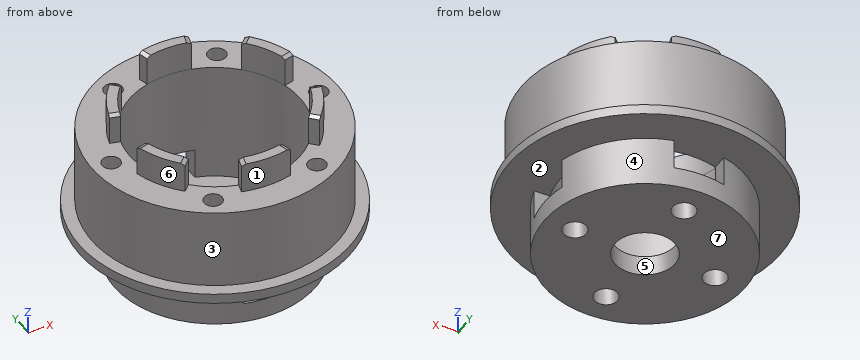
```python
from build123d import *
from OCP.BRepFilletAPI import BRepFilletAPI_MakeChamfer

# Parameters (mm, degrees)
SKETCH_1_R               = 10
EXTRUDE_1_DEPTH          = 2
SKETCH_2_R               = 10
SKETCH_2_R_2             = 8.5
EXTRUDE_2_DEPTH          = 3
SKETCH_4_R               = 13.5
SKETCH_4_R_2             = 8.5
EXTRUDE_3_DEPTH          = 1
SKETCH_5_R               = 12.25
SKETCH_5_R_2             = 8.5
EXTRUDE_4_DEPTH          = 8
SKETCH_6_R               = 0.9
CUT_EXTRUDE_1_DEPTH      = 8
SKETCH_7_R               = 3
SKETCH_7_R_2             = 1.15
CUT_EXTRUDE_2_DEPTH      = 24.674881204
CUT_EXTRUDE_3_DEPTH      = 24.674881204
CUT_EXTRUDE_3_DEPTH_BACK = 24.674881204
SKETCH_8_W               = 5
SKETCH_8_H               = 3
CUT_EXTRUDE_4_DEPTH      = 24.674881204
CUT_EXTRUDE_4_DEPTH_BACK = 24.674881204
SKETCH_9_W               = 3
SKETCH_9_H               = 5
EXTRUDE_5_DEPTH          = 3
CHAMFER_1_SIZE           = 0.2
CHAMFER_1_SIZE2          = 0.410060768


with BuildPart() as part:
    # 스케치1 → 보스-돌출1 (new body)
    with BuildSketch(Plane.XY):
        Circle(SKETCH_1_R)
    extrude(amount=EXTRUDE_1_DEPTH)

    # 스케치2 → 보스-돌출2 (add)
    with BuildSketch(Plane.XY.offset(2)):
        Circle(SKETCH_2_R)
        Circle(SKETCH_2_R_2, mode=Mode.SUBTRACT)
    extrude(amount=EXTRUDE_2_DEPTH)

    # 스케치4 → 보스-돌출3 (add)
    with BuildSketch(Plane.XY.offset(5)):
        Circle(SKETCH_4_R)
        Circle(SKETCH_4_R_2, mode=Mode.SUBTRACT)
    extrude(amount=EXTRUDE_3_DEPTH)

    # 스케치5 → 보스-돌출4 (add)
    with BuildSketch(Plane.XY.offset(6)):
        Circle(SKETCH_5_R)
        Circle(SKETCH_5_R_2, mode=Mode.SUBTRACT)
    extrude(amount=EXTRUDE_4_DEPTH)

    # 스케치6 → 컷-돌출1 (cut)
    with BuildSketch(Plane.XY.offset(14)):
        with Locations((10.375, 0)):
            Circle(SKETCH_6_R)
        with Locations((5.1875, -8.985013564)):
            Circle(SKETCH_6_R)
        with Locations((-5.1875, -8.985013564)):
            Circle(SKETCH_6_R)
        with Locations((-10.375, 0)):
            Circle(SKETCH_6_R)
        with Locations((-5.1875, 8.985013564)):
            Circle(SKETCH_6_R)
        with Locations((5.1875, 8.985013564)):
            Circle(SKETCH_6_R)
    extrude(amount=-CUT_EXTRUDE_1_DEPTH, mode=Mode.SUBTRACT)

    # 스케치7 → 컷-돌출2 (cut, through all)
    with BuildSketch(Plane(origin=(0, 0, 0), x_dir=(-1, 0, 0), z_dir=(0, 0, -1))):
        Circle(SKETCH_7_R)
        with Locations((-7, 0)):
            Circle(SKETCH_7_R_2)
        with Locations((7, 0)):
            Circle(SKETCH_7_R_2)
        with Locations((0, 7)):
            Circle(SKETCH_7_R_2)
        with Locations((0, -7)):
            Circle(SKETCH_7_R_2)
    extrude(amount=-CUT_EXTRUDE_2_DEPTH, mode=Mode.SUBTRACT)

    # 스케치8 → 컷-돌출3 (cut, two sides: drawn at the far end of the back side and taken through both)
    with BuildSketch(Plane(origin=(0, 0, 0), x_dir=(1, 0, 0), z_dir=(0, 1, 0)).offset(-CUT_EXTRUDE_3_DEPTH_BACK)):
        with Locations((0, -3.5)):
            Rectangle(SKETCH_8_W, SKETCH_8_H)
    extrude(amount=CUT_EXTRUDE_3_DEPTH + CUT_EXTRUDE_3_DEPTH_BACK, mode=Mode.SUBTRACT)

    # 스케치9 → 컷-돌출4 (cut, two sides: drawn at the far end of the back side and taken through both)
    with BuildSketch(Plane(origin=(0, 0, 0), x_dir=(0, 0, -1), z_dir=(1, 0, 0)).offset(-CUT_EXTRUDE_4_DEPTH_BACK)):
        with Locations((-3.5, 0)):
            Rectangle(SKETCH_9_W, SKETCH_9_H)
    extrude(amount=CUT_EXTRUDE_4_DEPTH + CUT_EXTRUDE_4_DEPTH_BACK, mode=Mode.SUBTRACT)

    # 스케치10 → 보스-돌출5 (add)
    with BuildSketch(Plane.XY.offset(14)):
        with BuildLine():
            Line((2.199961883, 8.210369523), (2.458780928, 9.17629535))
            ThreePointArc((2.458780928, 9.17629535), (0, 9.5), (-2.458780928, 9.17629535))
            Line((-2.458780928, 9.17629535), (-2.199961883, 8.210369523))
            ThreePointArc((-2.199961883, 8.210369523), (0, 8.5), (2.199961883, 8.210369523))
        make_face()
        with BuildLine():
            Line((6.01040764, 6.01040764), (6.717514421, 6.717514421))
            ThreePointArc((6.717514421, 6.717514421), (8.227241336, 4.75), (9.17629535, 2.458780928))
            Line((9.17629535, 2.458780928), (8.210369523, 2.199961883))
            ThreePointArc((8.210369523, 2.199961883), (7.361215932, 4.25), (6.01040764, 6.01040764))
        make_face()
        with BuildLine():
            Line((8.210369523, -2.199961883), (9.17629535, -2.458780928))
            ThreePointArc((9.17629535, -2.458780928), (8.227241336, -4.75), (6.717514421, -6.717514421))
            Line((6.717514421, -6.717514421), (6.01040764, -6.01040764))
            ThreePointArc((6.01040764, -6.01040764), (7.361215932, -4.25), (8.210369523, -2.199961883))
        make_face()
        with BuildLine():
            Line((2.199961883, -8.210369523), (2.458780928, -9.17629535))
            ThreePointArc((2.458780928, -9.17629535), (0, -9.5), (-2.458780928, -9.17629535))
            Line((-2.458780928, -9.17629535), (-2.199961883, -8.210369523))
            ThreePointArc((-2.199961883, -8.210369523), (0, -8.5), (2.199961883, -8.210369523))
        make_face()
        with BuildLine():
            Line((-6.01040764, -6.01040764), (-6.717514421, -6.717514421))
            ThreePointArc((-6.717514421, -6.717514421), (-8.227241336, -4.75), (-9.17629535, -2.458780928))
            Line((-9.17629535, -2.458780928), (-8.210369523, -2.199961883))
            ThreePointArc((-8.210369523, -2.199961883), (-7.361215932, -4.25), (-6.01040764, -6.01040764))
        make_face()
        with BuildLine():
            Line((-8.210369523, 2.199961883), (-9.17629535, 2.458780928))
            ThreePointArc((-9.17629535, 2.458780928), (-8.227241336, 4.75), (-6.717514421, 6.717514421))
            Line((-6.717514421, 6.717514421), (-6.01040764, 6.01040764))
            ThreePointArc((-6.01040764, 6.01040764), (-7.361215932, 4.25), (-8.210369523, 2.199961883))
        make_face()
    extrude(amount=EXTRUDE_5_DEPTH)

    # 모따기1: one chamfer whose edges measure the first distance from different faces: ONE call of the kernel's chamfer builder (chamfer() names one face for all edges)
    chamfer_1_edges_1 = [part.edges().sort_by_distance(p)[0] for p in [
        (-6.363961031, 6.363961031, 17),
    ]]
    chamfer_1_side_1 = [part.faces().sort_by_distance(p)[0] for p in [
        (-6.363961031, 6.363961031, 15.5),
    ]]
    chamfer_1_edges_2 = [part.edges().sort_by_distance(p)[0] for p in [
        (-8.693332437, 2.329371406, 17),
    ]]
    chamfer_1_side_2 = [part.faces().sort_by_distance(p)[0] for p in [
        (-8.693332437, 2.329371406, 15.5),
    ]]
    chamfer_1_edges_3 = [part.edges().sort_by_distance(p)[0] for p in [
        (-8.693332437, -2.329371406, 17),
    ]]
    chamfer_1_side_3 = [part.faces().sort_by_distance(p)[0] for p in [
        (-8.693332437, -2.329371406, 15.5),
    ]]
    chamfer_1_edges_4 = [part.edges().sort_by_distance(p)[0] for p in [
        (-6.363961031, -6.363961031, 17),
    ]]
    chamfer_1_side_4 = [part.faces().sort_by_distance(p)[0] for p in [
        (-6.363961031, -6.363961031, 15.5),
    ]]
    chamfer_1_edges_5 = [part.edges().sort_by_distance(p)[0] for p in [
        (-2.329371406, 8.693332437, 17),
    ]]
    chamfer_1_side_5 = [part.faces().sort_by_distance(p)[0] for p in [
        (-2.329371406, 8.693332437, 15.5),
    ]]
    chamfer_1_edges_6 = [part.edges().sort_by_distance(p)[0] for p in [
        (2.329371406, 8.693332437, 17),
    ]]
    chamfer_1_side_6 = [part.faces().sort_by_distance(p)[0] for p in [
        (2.329371406, 8.693332437, 15.5),
    ]]
    chamfer_1_edges_7 = [part.edges().sort_by_distance(p)[0] for p in [
        (-2.329371406, -8.693332437, 17),
    ]]
    chamfer_1_side_7 = [part.faces().sort_by_distance(p)[0] for p in [
        (-2.329371406, -8.693332437, 15.5),
    ]]
    chamfer_1_edges_8 = [part.edges().sort_by_distance(p)[0] for p in [
        (2.329371406, -8.693332437, 17),
    ]]
    chamfer_1_side_8 = [part.faces().sort_by_distance(p)[0] for p in [
        (2.329371406, -8.693332437, 15.5),
    ]]
    chamfer_1_edges_9 = [part.edges().sort_by_distance(p)[0] for p in [
        (6.363961031, 6.363961031, 17),
    ]]
    chamfer_1_side_9 = [part.faces().sort_by_distance(p)[0] for p in [
        (6.363961031, 6.363961031, 15.5),
    ]]
    chamfer_1_edges_10 = [part.edges().sort_by_distance(p)[0] for p in [
        (8.693332437, 2.329371406, 17),
    ]]
    chamfer_1_side_10 = [part.faces().sort_by_distance(p)[0] for p in [
        (8.693332437, 2.329371406, 15.5),
    ]]
    chamfer_1_edges_11 = [part.edges().sort_by_distance(p)[0] for p in [
        (6.363961031, -6.363961031, 17),
    ]]
    chamfer_1_side_11 = [part.faces().sort_by_distance(p)[0] for p in [
        (6.363961031, -6.363961031, 15.5),
    ]]
    chamfer_1_edges_12 = [part.edges().sort_by_distance(p)[0] for p in [
        (8.693332437, -2.329371406, 17),
    ]]
    chamfer_1_side_12 = [part.faces().sort_by_distance(p)[0] for p in [
        (8.693332437, -2.329371406, 15.5),
    ]]
    chamfer_1 = BRepFilletAPI_MakeChamfer(part.part.solid().wrapped)
    for e in chamfer_1_edges_1:
        chamfer_1.Add(CHAMFER_1_SIZE, CHAMFER_1_SIZE2, e.wrapped, chamfer_1_side_1[0].wrapped)  # the first distance lies on this face
    for e in chamfer_1_edges_2:
        chamfer_1.Add(CHAMFER_1_SIZE, CHAMFER_1_SIZE2, e.wrapped, chamfer_1_side_2[0].wrapped)  # the first distance lies on this face
    for e in chamfer_1_edges_3:
        chamfer_1.Add(CHAMFER_1_SIZE, CHAMFER_1_SIZE2, e.wrapped, chamfer_1_side_3[0].wrapped)  # the first distance lies on this face
    for e in chamfer_1_edges_4:
        chamfer_1.Add(CHAMFER_1_SIZE, CHAMFER_1_SIZE2, e.wrapped, chamfer_1_side_4[0].wrapped)  # the first distance lies on this face
    for e in chamfer_1_edges_5:
        chamfer_1.Add(CHAMFER_1_SIZE, CHAMFER_1_SIZE2, e.wrapped, chamfer_1_side_5[0].wrapped)  # the first distance lies on this face
    for e in chamfer_1_edges_6:
        chamfer_1.Add(CHAMFER_1_SIZE, CHAMFER_1_SIZE2, e.wrapped, chamfer_1_side_6[0].wrapped)  # the first distance lies on this face
    for e in chamfer_1_edges_7:
        chamfer_1.Add(CHAMFER_1_SIZE, CHAMFER_1_SIZE2, e.wrapped, chamfer_1_side_7[0].wrapped)  # the first distance lies on this face
    for e in chamfer_1_edges_8:
        chamfer_1.Add(CHAMFER_1_SIZE, CHAMFER_1_SIZE2, e.wrapped, chamfer_1_side_8[0].wrapped)  # the first distance lies on this face
    for e in chamfer_1_edges_9:
        chamfer_1.Add(CHAMFER_1_SIZE, CHAMFER_1_SIZE2, e.wrapped, chamfer_1_side_9[0].wrapped)  # the first distance lies on this face
    for e in chamfer_1_edges_10:
        chamfer_1.Add(CHAMFER_1_SIZE, CHAMFER_1_SIZE2, e.wrapped, chamfer_1_side_10[0].wrapped)  # the first distance lies on this face
    for e in chamfer_1_edges_11:
        chamfer_1.Add(CHAMFER_1_SIZE, CHAMFER_1_SIZE2, e.wrapped, chamfer_1_side_11[0].wrapped)  # the first distance lies on this face
    for e in chamfer_1_edges_12:
        chamfer_1.Add(CHAMFER_1_SIZE, CHAMFER_1_SIZE2, e.wrapped, chamfer_1_side_12[0].wrapped)  # the first distance lies on this face
    add(Compound.cast(chamfer_1.Shape()), mode=Mode.REPLACE)


solid = part.part
```
Design review of the part built by this model. Coordinates are the model's own, in mm. Face numbers are marked on the shaded views. A direction names the side the tool comes from. Give positions to 0.01 mm unless a question says otherwise; leave off trailing zeros. Order: outer loops, then holes, each group sorted by start corner. A loop starts at its lowest first (then second) coordinate and runs counter-clockwise, first axis right, second up. Notation, with made-up numbers: (80.25, -38) - (104.25, -38) arc R19 cw to (104.25, -15) - close; hole circle Ø3 at (74.25, 24.5). An arc over 180 degrees is marked (long way). Use a Markdown table: item, result. Add a question column.
(1) Add section A-A on z = 15. Give the boundary of the cut face in (x, y).
(2) Mouldability with a two-part tool opening along Y and no side actions: class the marked faces 4, 5, 6 and 7 as +Y half, -Y half, draft (parallel to the pull), parting line (faces both ways), or undercut.
(3) Add section B-B on z = 2.5. Give the boundary of the cut face in (x, y), then the cut area to 3 significant figures.
(4) Add section C-C on x = -0.25. Give the number of separate pieces and of enclosed holes in the cut face, then the cut area to 3 significant figures.
(5) Machinability: for the marked faces 1, 2 and 3, which of the approach directions +Z, -Z, +X, -X, +Y, -Y give a long, thin tool a straight path to every point of the face, cutting with its end or side? Answer none if there is none.
(6) Wall thickness on probe 1 along Y at (x, z) = (0, 0.55); probe 2 along Z at (x, y) = (9, -0.25); probe 3 along Y at (x, z) = (5.75, 6.75): over which ranges is each line inside the solid? List them lowest first. Write a range as [from, to].
(7) Clearance check with flat-ended pins moving along their axes: P1, Ø0.9, axis at x = -10, y = 0.5, coming from the +Z side; P2, Ø1.7, axis at x = -9, z = 3.5, coming from the +Y side; P3, Ø1, axis at x = -5, z = 9, coming from the +Y side; P4, Ø1.4, axis at x = -7, y = 0, coming from the +Z side. State where each tip first meets the part, or that it passes through.
Report:
| question | item | result |
|---|---|---|
| 1 | outline | (-9.18, -2.46) arc R9.5 ccw to (-6.72, -6.72) - (-6.01, -6.01) arc R8.5 cw to (-8.21, -2.2) - close; (-9.18, 2.46) - (-8.21, 2.2) arc R8.5 cw to (-6.01, 6.01) - (-6.72, 6.72) arc R9.5 ccw to start; (-2.46, -9.18) arc R9.5 ccw to (2.46, -9.18) - (2.2, -8.21) arc R8.5 cw to (-2.2, -8.21) - close; (-2.46, 9.18) - (-2.2, 8.21) arc R8.5 cw to (2.2, 8.21) - (2.46, 9.18) arc R9.5 ccw to start; (6.01, -6.01) - (6.72, -6.72) arc R9.5 ccw to (9.18, -2.46) - (8.21, -2.2) arc R8.5 cw to start; (6.01, 6.01) arc R8.5 cw to (8.21, 2.2) - (9.18, 2.46) arc R9.5 ccw to (6.72, 6.72) - close |
| 2 | face 4 | parting line |
| 2 | face 5 | undercut |
| 2 | face 6 | -Y half |
| 2 | face 7 | draft |
| 3 | outline | (-9.68, -2.5) arc R10 ccw to (-2.5, -9.68) - (-2.5, -8.12) arc R8.5 cw to (-8.12, -2.5) - close; (-9.68, 2.5) - (-8.12, 2.5) arc R8.5 cw to (-2.5, 8.12) - (-2.5, 9.68) arc R10 ccw to start; (2.5, -9.68) arc R10 ccw to (9.68, -2.5) - (8.12, -2.5) arc R8.5 cw to (2.5, -8.12) - close; (2.5, 8.12) arc R8.5 cw to (8.12, 2.5) - (9.68, 2.5) arc R10 ccw to (2.5, 9.68) - close |
| 3 | area | 56.8 mm² |
| 4 | separate pieces | 6 |
| 4 | enclosed holes | 0 |
| 4 | area | 95.1 mm² |
| 5 | face 1 | +Z, -Y |
| 5 | face 2 | none |
| 5 | face 3 | +Z |
| 6 | probe 1 | y = [-10, -8.15], [-5.85, -3], [3, 5.85], [8.15, 10] |
| 6 | probe 2 | z = [0, 2], [5, 14] |
| 6 | probe 3 | y = [-10.82, -9.69], [-8.28, -6.26], [6.26, 8.28], [9.69, 10.82] |
| 7 | P1 | stops at z = 14 |
| 7 | P2 | stops at y = 5.79 |
| 7 | P3 | stops at y = 11.39 |
| 7 | P4 | passes through |
